from build123d import *

# Parameters (mm, degrees)
F0_R     = 16.168204
F0_W     = 62.179334
F0_H     = 76.463766
F1_DEPTH = 22.352
F2_DEPTH = 43.18
F4_DEPTH = 25.4
F5_DEPTH = 25.4


with BuildPart() as f1:
    # F0 (on Front) → F1 (new body)
    with BuildSketch(Plane.XZ):
        Circle(F0_R)
        Rectangle(F0_W, F0_H)
        Circle(F0_R, mode=Mode.SUBTRACT)
    extrude(amount=F1_DEPTH)

    # F0 (on Front) → F2 (join)
    with BuildSketch(Plane.XZ):
        Circle(F0_R)
    extrude(amount=F2_DEPTH)

    # F3 (on Right) → F4 (cut)
    with BuildSketch(Plane.YZ):
        Polygon((-43.015767, 17.78225), (-58.439311, 18.220695), (-58.439311, -16.693853), (-23.446971, -16.693853), align=None)
    extrude(amount=F4_DEPTH, mode=Mode.SUBTRACT)

    # F3 (on Right) → F5 (cut)
    with BuildSketch(Plane.YZ):
        Polygon((-43.015767, 17.78225), (-58.439311, 18.220695), (-58.439311, -16.693853), (-23.446971, -16.693853), align=None)
    extrude(amount=-F5_DEPTH, mode=Mode.SUBTRACT)


solid = f1.part
Verification items for the finished model (mm, model axes). Coordinates: 2 decimals unless noted, no trailing zeros. Loops run counter-clockwise (first coordinate to the right, second up) from the corner with the lowest first, then second, coordinate; pieces in that order, holes last. Notation, with made-up numbers: M 72,5 L 110,5 A31 ccw 110,37 Z; hole C 12.5,83.25 d9. An arc over 180 degrees is marked long. One line per item, written item: value.
1. Mould release check, pull along Z, two halves, no side actions. Record for faces 1 (the flat face through (0, -11, -38.232)), 2 (the cylindrical face through (-2.1, -29.89, 16.03)), 3 (the flat face through (0, -11, 38.232)), 4 (the flat face through (0, 0, 1)): pulls with the +Z half, pulls with the -Z half, needs draft (parallel to the pull), parting line crosses it, or undercut.
Answers follow:
face 1: pulls with the -Z half
face 2: parting line crosses it
face 3: pulls with the +Z half
face 4: needs draft
2. Section check B-B on z = 8.5. Record the cut outline in (x, y), plus the area to 3 significant figures.
Answers follow:
outline: M -31.09,-22.35 L -13.75,-22.35 L -13.75,-37.75 L 13.75,-37.75 L 13.75,-22.35 L 31.09,-22.35 L 31.09,0 L -31.09,0 Z
area: 1,810 mm^2
3. Section check A-A on x = 0. Record the cut outline in (y, z), plus the area to 3 significant figures.
Answers follow:
outline: M -42.1,16.17 L -23.75,-16.17 L -22.35,-16.17 L -22.35,-38.23 L 0,-38.23 L 0,38.23 L -22.35,38.23 L -22.35,16.17 Z
area: 2,050 mm^2
4. Gauge pin test, flat end, axial feed: P1, Ø2, axis at x = 16.5, z = 30.5, coming from the -Y side. Record the tip position at first contact, or that the pin passes through.
Answers follow:
P1: y = -22.35
5. Section check D-D on x = 20.5. Record the cut outline in (y, z).
Answers follow:
outline: M -22.35,-38.23 L 0,-38.23 L 0,38.23 L -22.35,38.23 Z
6. Material ranges on line 1 along Y through (x, z) = (9, -35); line 2 along Z through (x, y) = (-6, -22.5); line 3 along Z through (x, y) = (6, -28.5), recorded low to high. Write a range as from..to.
Answers follow:
line 1: -22.35..0
line 2: -15.01..15.01
line 3: -7.79..15.01
7. Section check C-C on y = -25. Record the cut outline in (x, z), plus the area to 3 significant figures.
Answers follow:
outline: M -8.16,-13.96 L 8.16,-13.96 A16.17 ccw long Z
area: 797 mm^2
